```python
from build123d import *

# Parameters (mm, degrees)
SKETCH5_R               = 10.5
SKETCH5_R_2             = 9.2
BOSS_EXTRUDE1_DEPTH     = 15
SKETCH6_R               = 10.5
BOSS_EXTRUDE2_DEPTH     = 2
SKETCH7_W               = 2
SKETCH7_H               = 10
EXTRUDE_THIN1_DEPTH     = 10
SKETCH8_W               = 2
SKETCH8_H               = 9.64593802
EXTRUDE_THIN2_DEPTH     = 10
CUT_EXTRUDE1_DEPTH      = 29.456038339
CUT_EXTRUDE1_DEPTH_BACK = 29.456038339
SKETCH9_R               = 1


with BuildPart() as part:
    # Sketch5 → Boss-Extrude1 (new body)
    with BuildSketch(Plane.XY):
        Circle(SKETCH5_R)
        Circle(SKETCH5_R_2, mode=Mode.SUBTRACT)
    extrude(amount=BOSS_EXTRUDE1_DEPTH)

    # Sketch6 → Boss-Extrude2 (add)
    with BuildSketch(Plane.XY):
        Circle(SKETCH6_R)
    extrude(amount=BOSS_EXTRUDE2_DEPTH)

    # Sketch7 → Extrude-Thin1 (add)
    with BuildSketch(Plane(origin=(0, 0, 0), x_dir=(-1, 0, 0), z_dir=(0, 0, -1))):
        with Locations((-2, 15.062305899)):
            Rectangle(SKETCH7_W, SKETCH7_H)
    extrude(amount=-EXTRUDE_THIN1_DEPTH)

    # Sketch8 → Extrude-Thin2 (add)
    with BuildSketch(Plane(origin=(0, 0, 0), x_dir=(-1, 0, 0), z_dir=(0, 0, -1))):
        with Locations((2, 14.885274909)):
            Rectangle(SKETCH8_W, SKETCH8_H)
    extrude(amount=-EXTRUDE_THIN2_DEPTH)

    # Sketch9 → Cut-Extrude1 (cut, two sides: drawn at the far end of the back side and taken through both)
    with BuildSketch(Plane.ZY.offset(3).offset(-CUT_EXTRUDE1_DEPTH_BACK)):
        with Locations((5, 13.45227248)):
            Circle(SKETCH9_R)
        with Locations((5, 18.45227248)):
            Circle(SKETCH9_R)
    extrude(amount=CUT_EXTRUDE1_DEPTH + CUT_EXTRUDE1_DEPTH_BACK, mode=Mode.SUBTRACT)


solid = part.part
```
The listing builds one solid part. Answer for the finished solid, in the listing's coordinates (mm). A direction names the side the tool comes from. Give positions to 0.01 mm unless a question says otherwise; leave off trailing zeros. Loops run counter-clockwise (first coordinate to the right, second up) from the corner with the lowest first, then second, coordinate; pieces in that order, holes last. Notation, with made-up numbers: (22.5, 78) - (46.5, 78) arc R23 ccw to (46.5, 94) - close; hole circle Ø11 at (87.25, -21). An arc over 180 degrees is marked (long way). Return JSON: item names as keys, results as strings. Group by question number.
1. Find section D-D (x = 0). Write down the section's boundary in (y, z), then the cut area to 3 significant figures.
2. Find section B-B (y = 12). Write down the section's boundary in (x, z).
3. Find section C-C (z = 7.75). Write down the section's boundary in (x, y), then the cut area to 3 significant figures.
4. Which of the six approach directions +Z, -Z, +X, -X, +Y, -Y give full straight-line access (tool end or side, diameter ignored) to faces 1 (the cylindrical face through (-7.3, -5.6, 8.4)), 2 (the flat face through (3, 15, 5)), 3 (the flat face through (-2, 19.708, 5))?
5. Determine the mould class of faces 4 (the flat face through (-3, 15, 5)), 5 (the flat face through (6.2, -7, 15)), 6 (the flat face through (0, 0, 2)) for opening direction X: pulls with the +X half, pulls with the -X half, needs draft (parallel to the pull), parting line crosses it, or undercut.
6. Find section A-A (z = 5). Write down the section's boundary in (x, y).
7. Given pin 1 Ø5 at (y, z) = (13.5, 4) entering from -X; pin 2 Ø2 at (x, z) = (-2, 6.5) entering from +Y; pin 3 Ø3 at (y, z) = (16, 4.5) entering from +X, each flat-ended and moving along its own axis, determine where each tip first touches the part or whether it passes through.
8. Straight lines are drawn through the part: line 1 (Y direction, x = 0, z = 10); line 2 (Y direction, x = -2, z = 4.5); line 3 (Y direction, x = 2, z = 5). For each, find the intervals that lie inside material, in ascending order. Write a range as [from, to].
Verdict:
{
 "1": {"outline": "(-10.5, 0) - (10.5, 0) - (10.5, 15) - (9.2, 15) - (9.2, 2) - (-9.2, 2) - (-9.2, 15) - (-10.5, 15) - close", "area": "75.8 mm^2"},
 "2": {"outline": "(-3, 0) - (-1, 0) - (-1, 10) - (-3, 10) - close; (1, 0) - (3, 0) - (3, 10) - (1, 10) - close"},
 "3": {"outline": "(-3, 10.06) arc R10.5 ccw (long way) to (3, 10.06) - (3, 20.06) - (1, 20.06) - (1, 10.45) arc R10.5 ccw to (-1, 10.45) - (-1, 19.71) - (-3, 19.71) - close; hole circle Ø18.4 at (0, 0)", "area": "119 mm^2"},
 "4": {"face 1": "+Z", "face 2": "+Z, -Z, +X, +Y", "face 3": "+Z, -Z, -X, +Y"},
 "5": {"face 4": "pulls with the -X half", "face 5": "needs draft", "face 6": "undercut"},
 "6": {"outline": "(-3, 10.06) arc R10.5 ccw (long way) to (3, 10.06) - (3, 12.45) - (1, 12.45) - (1, 10.45) arc R10.5 ccw to (-1, 10.45) - (-1, 12.45) - (-3, 12.45) - close; (-3, 14.45) - (-1, 14.45) - (-1, 17.45) - (-3, 17.45) - close; (-3, 19.45) - (-1, 19.45) - (-1, 19.71) - (-3, 19.71) - close; (1, 14.45) - (3, 14.45) - (3, 17.45) - (1, 17.45) - close; (1, 19.45) - (3, 19.45) - (3, 20.06) - (1, 20.06) - close; hole circle Ø18.4 at (0, 0)"},
 "7": {"pin 1": "stops at x = -3", "pin 2": "stops at y = 19.71", "pin 3": "stops at x = 3"},
 "8": {"line 1": "y = [-10.5, -9.2], [9.2, 10.5]", "line 2": "y = [-10.31, -8.98], [8.98, 12.59], [14.32, 17.59], [19.32, 19.71]", "line 3": "y = [-10.31, -8.98], [8.98, 12.45], [14.45, 17.45], [19.45, 20.06]"}
}
